The listing builds one solid part. Answer for the finished solid, in the listing's coordinates (mm). A direction names the side the tool comes from. Give positions to 0.01 mm unless a question says otherwise; leave off trailing zeros. Order: outer loops, then holes, each group sorted by start corner. A loop starts at its lowest first (then second) coordinate and runs counter-clockwise, first axis right, second up. Notation, with made-up numbers: (47, 21.25) - (89, 21.25) arc R13 ccw to (89, 43.25) - close; hole circle Ø9 at (27, -9). An arc over 180 degrees is marked (long way). Use a Markdown table: item, result. Add a question column.
1) Find section B-B, the plane y = 3. Determine the outline of the cut face in (x, z), plus the area to 3 significant figures.
2) Flat-ended cylindrical pins translate along their axes: pin 1 (1.4 mm diameter, centred on x = 207.5, z = 0, fed in from +Y); pin 2 (1.5 mm diameter, centred on x = 209.5, z = 0, fed in from +Y); pin 3 (0.6 mm diameter, centred on x = 207, z = 0, fed in from -Y). Find the tip coordinate at first contact, or state that the pin passes through.
3) Straight lines are drawn through the part: line 1 (Y direction, x = 202.5, z = -1.3); line 2 (Y direction, x = 197, z = 0.5); line 3 (X direction, y = 7, z = -0.9). For each, find the intervals that lie inside material, in ascending order.
4) Find section A-A, the plane x = 195. Determine the outline of the cut face in (y, z).
5) The mould has two halves that part along X. Classify faces 1 (the face through (205.5, -1, 0)), 2 (the face through (221.5, -1, 0)), 3 (the face through (202, -3, 0)), 4 (the face through (195.5, 25, 0)): released by +X, released by -X, zero draft, split by the parting line, or undercut.
6) Find section D-D, the plane y = 15.5. Determine the outline of the cut face in (x, z).
7) Find section C-C, the plane x = 216. Determine the outline of the cut face in (y, z).
8) For faces 5 (the face through (205.07, -2.55, 0.02)), 6 (the face through (207, 6.3, 0)), 7 (the face through (198, 23.5, 0)), 8 (the face through (194, 34, 0)), 9 (the face through (223, 0, 0)), determine the directions among +Z, -Z, +X, -X, +Y, -Y from which every point of the face is accessible in a straight line to the end or side of a thin tool.
from build123d import *

# Parameters (mm, degrees)
PAD007_DEPTH = 3
FILLET011_R  = 6
FILLET012_R  = 1.5


with BuildPart() as part:
    # Sketch006 → Pad007 (new body)
    with BuildSketch(Plane(origin=(195.5, 0, -1.5), x_dir=(1, 0, 0), z_dir=(0, 0, 1))):
        Polygon((0, 36), (12, 36), (28, 12), (28, 0), (26, 0), (26, -3), (18, -3), (18, 0), (15.5, 0), (15.5, 4), (16.75, 4), (16.75, 6.3), (15.5, 6.3), (15.5, 9.3), (12.5, 9.3), (12.5, 6.3), (11.25, 6.3), (11.25, 4), (12.5, 4), (12.5, 0), (10, 0), (10, -3), (2, -3), (2, 0), (0, 0), (0, 10), (-3, 10), (-3, 18), (0, 18), (0, 20.5), (4, 20.5), (4, 19.25), (6.3, 19.25), (6.3, 20.5), (9.3, 20.5), (9.3, 23.5), (6.3, 23.5), (6.3, 24.75), (4, 24.75), (4, 23.5), (0, 23.5), (0, 26), (-3, 26), (-3, 34), (0, 34), align=None)
    extrude(amount=PAD007_DEPTH)

    # Fillet011
    fillet011_edges = [part.edges().sort_by_distance(p)[0] for p in [
        (207.5, 36, 0),
        (223.5, 12, 0),
    ]]
    fillet(fillet011_edges, radius=FILLET011_R)

    # Fillet012
    fillet012_edges = [part.edges().sort_by_distance(p)[0] for p in [
        (221.5, -3, 0),
        (213.5, -3, 0),
        (205.5, -3, 0),
        (197.5, -3, 0),
    ]]
    fillet(fillet012_edges, radius=FILLET012_R)


solid = part.part
The answers:
| question | item | result |
|---|---|---|
| 1 | outline | (195.5, -1.5) - (208, -1.5) - (208, 1.5) - (195.5, 1.5) - close; (211, -1.5) - (223.5, -1.5) - (223.5, 1.5) - (211, 1.5) - close |
| 1 | area | 75.0 mm2 |
| 2 | pin 1 | y = 35.45 |
| 2 | pin 2 | y = 34.01 |
| 2 | pin 3 | y = 0 |
| 3 | line 1 | -3 to 20.5, 23.5 to 36 |
| 3 | line 2 | 0 to 20.5, 23.5 to 36 |
| 3 | line 3 | 195.5 to 208, 211 to 223.5 |
| 4 | outline | (10, -1.5) - (18, -1.5) - (18, 1.5) - (10, 1.5) - close; (26, -1.5) - (34, -1.5) - (34, 1.5) - (26, 1.5) - close |
| 5 | face 1 | undercut |
| 5 | face 2 | released by +X |
| 5 | face 3 | zero draft |
| 5 | face 4 | released by -X |
| 6 | outline | (192.5, -1.5) - (221.17, -1.5) - (221.17, 1.5) - (192.5, 1.5) - close |
| 7 | outline | (-3, -1.5) - (23.25, -1.5) - (23.25, 1.5) - (-3, 1.5) - close |
| 8 | face 5 | +Z, -Z, -Y |
| 8 | face 6 | +Z, -Z |
| 8 | face 7 | +Z, -Z, -X |
| 8 | face 8 | +Z, -Z, -X, +Y |
| 8 | face 9 | +Z, -Z, +X, -Y |
